Model file for the job. Use its own axes, mm. A direction names the side the tool comes from. Give positions to 0.01 mm unless a question says otherwise; leave off trailing zeros. Loops run counter-clockwise (first coordinate to the right, second up) from the corner with the lowest first, then second, coordinate; pieces in that order, holes last. Notation, with made-up numbers: M -39,-6.75 L -10,-6.75 A14 ccw -10,14.25 Z; hole C 45,-30 d8. An arc over 180 degrees is marked long. Answer in a Markdown table with one row per item.
```python
from build123d import *

# Parameters (mm, degrees)
BOSS_EXTRUDE1_DEPTH = 10
SKETCH10_R          = 1.5
CUT_EXTRUDE9_DEPTH  = 20
SKETCH11_R          = 1.730599661
CUT_EXTRUDE10_DEPTH = 112.446287057
SKETCH12_R          = 5
BOSS_EXTRUDE4_DEPTH = 20
CUT_EXTRUDE11_START = -10.000002096
CUT_EXTRUDE11_DEPTH = 10.000002096
SKETCH14_R          = 2
CUT_EXTRUDE12_DEPTH = 71.851658179
CHAMFER1_SIZE       = 0.5


# Read off the part's stored shape, not the designer's step: Cut-Extrude11
with BuildPart() as part:
    # Sketch1 → Boss-Extrude1 (new body)
    with BuildSketch(Plane.XY):
        Polygon((51.23475383, 0), (51.23475383, 21.423100566), (9.462915873, 42.664679757), (-9.462915873, 42.664679757), (-51.23475383, 21.423100566), (-51.23475383, 0), align=None)
    extrude(amount=BOSS_EXTRUDE1_DEPTH)

    # Sketch10 → Cut-Extrude9 (cut)
    with BuildSketch(Plane(origin=(0, 0, 0), x_dir=(-1, 0, 0), z_dir=(0, 0, -1))):
        with Locations((0, 21.332339879)):
            Circle(SKETCH10_R)
        with Locations((10, 21.332339879)):
            Circle(SKETCH10_R)
        with Locations((20, 21.332339879)):
            Circle(SKETCH10_R)
        with Locations((30, 21.332339879)):
            Circle(SKETCH10_R)
        with Locations((-10, 21.332339879)):
            Circle(SKETCH10_R)
        with Locations((-20, 21.332339879)):
            Circle(SKETCH10_R)
        with Locations((-30, 21.332339879)):
            Circle(SKETCH10_R)
        with Locations((10, 12.332339879)):
            Circle(SKETCH10_R)
        with Locations((0, 12.332339879)):
            Circle(SKETCH10_R)
        with Locations((20, 12.332339879)):
            Circle(SKETCH10_R)
        with Locations((30, 12.332339879)):
            Circle(SKETCH10_R)
        with Locations((-10, 12.332339879)):
            Circle(SKETCH10_R)
        with Locations((-20, 12.332339879)):
            Circle(SKETCH10_R)
        with Locations((-30, 12.332339879)):
            Circle(SKETCH10_R)
    extrude(amount=-CUT_EXTRUDE9_DEPTH, mode=Mode.SUBTRACT)

    # Sketch11 → Cut-Extrude10 (cut, through all)
    with BuildSketch(Plane(origin=(51.23475383, 0, 0), x_dir=(0, 0, -1), z_dir=(1, 0, 0))):
        with Locations(Location((-5, 7.5, 0), (0, 0, 90))):
            Circle(SKETCH11_R)
    extrude(amount=-CUT_EXTRUDE10_DEPTH, mode=Mode.SUBTRACT)

    # Sketch12 → Boss-Extrude4 (add)
    with BuildSketch(Plane.XY.offset(10)):
        with Locations((0, 33.664679757)):
            Circle(SKETCH12_R)
    extrude(amount=BOSS_EXTRUDE4_DEPTH)

    # Cut-Extrude11 outline → Cut-Extrude11 (cut)
    with BuildSketch(Plane(origin=(5, 0, 0), x_dir=(0, 0, -1), z_dir=(1, 0, 0)).offset(CUT_EXTRUDE11_START)):
        with BuildLine():
            ThreePointArc((-22, 30.665551075), (-19.000871318, 33.664679757), (-22, 36.663808439))
            Line((-22, 36.663808439), (-22, 36.664679757))
            Line((-22, 36.664679757), (-30, 36.664679757))
            Line((-30, 36.664679757), (-30, 30.664679757))
            Line((-30, 30.664679757), (-22, 30.664679757))
            Line((-22, 30.664679757), (-22, 30.665551075))
        make_face()
    extrude(amount=CUT_EXTRUDE11_DEPTH, mode=Mode.SUBTRACT)

    # Sketch14 → Cut-Extrude12 (cut, through all)
    with BuildSketch(Plane(origin=(0, 38.664679757, 0), x_dir=(1, 0, 0), z_dir=(0, 1, 0))):
        with Locations(Location((0, -26, 0), (0, 0, 270))):
            Circle(SKETCH14_R)
        Polygon((-4.00065334, -22), (-1, -30), (-4, -30), align=None)
        Polygon((1, -30), (4, -30), (4.00065334, -22), align=None)
    extrude(amount=-CUT_EXTRUDE12_DEPTH, mode=Mode.SUBTRACT)

    # Chamfer1
    chamfer1_edges = [part.edges().sort_by_distance(p)[0] for p in [
        (1, 29.715190014, 30),
        (1, 37.6141695, 30),
        (0, 36.664679757, 30),
        (0, 28.664679757, 30),
        (0, 38.664679757, 30),
        (0, 30.664679757, 30),
        (-1, 29.715190014, 30),
        (-1, 37.6141695, 30),
    ]]
    chamfer(chamfer1_edges, length=CHAMFER1_SIZE)


solid = part.part
```
(1) Flat gauge pins, fed straight in: P1, Ø2, axis at x = -0.5, z = 25, coming from the -Y side; P2, Ø6, axis at x = -22, z = 4, coming from the -Y side; P3, Ø3, axis at x = -14.5, y = 35, coming from the +Z side; P4, Ø2, axis at x = 34.5, z = 4, coming from the +Y side. Where does each tip first touch, or does it go through?
Established:
| item | result |
|---|---|
| P1 | stops at y = 28.67 |
| P2 | stops at y = 0 |
| P3 | stops at z = 10 |
| P4 | stops at y = 30.44 |
(2) Saw through at B-B, the plane z = 5. Count the separate pieces of the cut face and the enclosed holes in it, and give its area (3 significant figures).
Established:
| item | result |
|---|---|
| separate pieces | 2 |
| enclosed holes | 14 |
| area | 3,030 mm2 |
(3) Which spindle directions (+Z, -Z, +X, -X, +Y, -Y) get a long thin tool onto all of the face, cutting with end or side? Do faces 1 (the flat face through (1, 36.665, 24)), 2 (the flat face through (2.294, 37.4, 26.551)). Say none if no direction does.
Established:
| item | result |
|---|---|
| face 1 | +Z, +X, -X |
| face 2 | +Z, +X, +Y, -Y |
(4) Wall check: L1, parallel to Z at x = 0, y = 37.6; L2, parallel to Z at x = -13.5, y = 13.5; L3, parallel to Y at x = 10, z = 7.5. Give the ranges that are in metal, low to high.
Established:
| item | result |
|---|---|
| L1 | z = 0 to 24, 28 to 30 |
| L2 | z = 0 to 10 |
| L3 | y = 0 to 10.83, 13.83 to 19.83, 22.83 to 42.39 |
(5) Saw through at D-D, the plane z = 26. Give the cut face in (x, y), and give its area (3 significant figures).
Established:
| item | result |
|---|---|
| outline | M -2.5,29.33 A5 ccw -2,29.08 L -2,30.66 L -2.5,30.66 Z; M -2.5,36.66 L -2,36.66 L -2,38.25 A5 ccw -2.5,37.99 Z; M 2,29.08 A5 ccw 2.5,29.33 L 2.5,30.66 L 2,30.66 Z; M 2,36.66 L 2.5,36.66 L 2.5,37.99 A5 ccw 2,38.25 Z |
| area | 2.93 mm2 |
(6) Mould opens along Y. For faces 3 (the cylindrical face through (-1.084, 28.784, 17.447)), 4 (the flat face through (0, 42.665, 5)), 5 (the flat face through (-51.235, 11, 5)), 6 (the cylindrical face through (0.33, 10.87, 4.93)) say: pulls with the +Y half, pulls with the -Y half, needs draft (parallel to the pull), parting line crosses it, or undercut.
Established:
| item | result |
|---|---|
| face 3 | parting line crosses it |
| face 4 | pulls with the +Y half |
| face 5 | needs draft |
| face 6 | undercut |
(7) Saw through at C-C, the plane y = 7.5. Give the cut face in (x, z).
Established:
| item | result |
|---|---|
| outline | M -51.23,0 L 51.23,0 L 51.23,3.27 L -51.23,3.27 Z; M -51.23,6.73 L 51.23,6.73 L 51.23,10 L -51.23,10 Z |
(8) Saw through at A-A, the plane x = -30. Give the cut face in (y, z), and give its area (3 significant figures).
Established:
| item | result |
|---|---|
| outline | M 0,0 L 10.83,0 L 10.83,10 L 0,10 Z; M 13.83,0 L 19.83,0 L 19.83,10 L 13.83,10 Z; M 22.83,0 L 32.22,0 L 32.22,10 L 22.83,10 Z; hole C 7.5,5 d3.46 |
| area | 253 mm2 |
